Autodesk Inventor part; units mm, degrees
ref_plane "Start Plane" through (0, 0, 0) normal (0, 0, 1) x (1, 0, 0)
ref_plane "End Plane" through (0, 0, 105.4293) normal (0, 0, 1) x (1, 0, 0)
ref_plane "Work Plane4" through (163.4562, -7, -44.6771) normal (0.6544, 0, 0.7562) x (0.7562, 0, -0.6544)
ref_plane "Start Plane" through (0, 0, 0) normal (0, 0, 1) x (1, 0, 0)
ref_plane "End Plane" through (0, 0, 105.4293) normal (0, 0, 1) x (1, 0, 0)
sketch "Sketch" plane through (0, 0, 0) normal (0, 0, 1) x (1, 0, 0)
  line L0 (-10, -7) -> (-10, 7)
  line L1 (-7, 10) -> (7, 10)
  line L2 (10, 7) -> (10, -7)
  line L3 (7, -10) -> (-7, -10)
  arc A0 (-10, -7) -> (-7, -10) centre (-7, -7) ccw
  arc A1 (-7, 10) -> (-10, 7) centre (-7, 7) ccw
  arc A2 (10, 7) -> (7, 10) centre (7, 7) ccw
  arc A3 (7, -10) -> (10, -7) centre (7, -7) ccw
  arc A4 (-7, 8) -> (-8, 7) centre (-7, 7) ccw
  line L4 (-7, 8) -> (7, 8)
  arc A5 (8, 7) -> (7, 8) centre (7, 7) ccw
  line L5 (8, 7) -> (8, -7)
  arc A6 (7, -8) -> (8, -7) centre (7, -7) ccw
  line L6 (7, -8) -> (-7, -8)
  arc A7 (-8, -7) -> (-7, -8) centre (-7, -7) ccw
  line L7 (-8, -7) -> (-8, 7)
  line L8 (0, 14.8698) -> (0, -14.8698) construction
  line L9 (-14.8698, 0) -> (14.8698, 0) construction
  dimension "d7" = 3
  dimension "d10" = 20
  dimension "d11" = 20
  dimension "d12" = 2
  dimension "d15" = 10
  dimension "d16" = 10
extrude "Body" add sketch "Sketch" along normal up to surface (105.4293 mm away) from surface at 0
sketch "Sketch3" plane through (0, 0, 0) normal (0, 0, 1) x (1, 0, 0)
  line L0 (0, 0) -> (10, 0)
ref_plane "Work Plane3" through (0, 0, 0) normal (0, -1, 0) x (1, 0, 0)
sketch "Sketch4" plane through (0, 0, 0) normal (0, -1, 0) x (1, 0, 0)
  line L0 (-2, 0) -> (12, 0)
  line L1 (-2, 105.4293) -> (12, 105.4293)
  dimension "d18" = 105.4293
ref_plane "Work Plane4" through (163.4562, -7, -44.6771) normal (0.6544, 0, 0.7562) x (0.7562, 0, -0.6544)
split "Split1" plane through (163.4562, -7, -44.6771) removes the side toward (0.6544, 0, 0.7562)
sketch "Sketch9" plane through (-7, 10, 0) normal (0, 1, 0) x (1, 0, 0)
  line L0 (0, -102.8331) -> (-3, -105.4293)
  line L1 (-3, 0) -> (-3, -105.4293)
  line L2 (0, -102.8331) -> (14, -90.7177)
  line L3 (17, -88.1216) -> (14, -90.7177)
  line L4 (17, 0) -> (17, -88.1216)
  line L5 (0, 0) -> (14, 0)
  line L6 (0, 0) -> (-3, 0)
  line L7 (17, 0) -> (14, 0)
  line L8 (0.3719, -13.6065) -> (0.3719, -23.9385)
  line L9 (13.8719, -23.9385) -> (13.8719, -13.6065)
  circle A0 centre (7.1219, -18.7725) radius 8.5
  line L10 (14.1439, -13.9827) -> (14.1439, -23.5624)
  line L11 (0.2439, -23.7668) -> (0.2439, -13.7783)
  line L12 (14.1439, -13.9827) -> (14.1439, 0)
  line L13 (0.2439, -13.7783) -> (0.2439, 0)
  line L14 (17, 0) -> (17, -88.1216)
  line L15 (17, -67.4293) -> (-3, -67.4293)
  line L16 (-3, 0) -> (-3, -105.4293)
  line L17 (17, -86.1216) -> (-3, -86.1216)
  line L18 (14.1439, -23.5624) -> (14.1439, -27.2725)
  line L19 (14.1439, -27.2725) -> (0.2439, -27.2725)
  line L20 (0.2439, -27.2725) -> (0.2439, -23.7668)
  line L21 (17, -8) -> (-3, -8)
  point P0 (7, 0)
  point P1 (7.117, -27.2725)
  point P2 (14.1439, -7.7933)
  point P3 (17, -67.4293)
  point P4 (-3, -67.4293)
  point P5 (0.2439, -7.7933)
  point P6 (7.1219, -27.2725)
  point P7 (0.2439, -8)
  point P8 (14.1439, -8)
  point P9 (14.1439, -8)
  point P10 (0.2439, -8)
  dimension "d44" = 13.5
  dimension "d45" = 13.9
  dimension "d47" = 2
  dimension "d49" = 38
  dimension "d53" = 8
extrude "Extrusion8" cut sketch "Sketch9" against normal through all contours L1 L6 L5 L13 L21 | L21 L12 A0 L13 | L13 L5 L7 L12 L21 | L21 L12 L7 L4 | A0 L8 L11 | A0 L9 L8 | A0 L19 L20 | L10 A0 L9 | L18 L19 A0
equation "\"d7\" = G_IR"
equation "\"d10\" = G_H"
equation "\"d11\" = G_W"
equation "\"d12\" = G_T"
equation "\"d15\" = 0.5 * d10"
equation "\"d16\" = 0.5 * d11"
equation "\"d3\" = G_L"
equation "\"G_W\" = 20"
equation "\"G_H\" = 20"
equation "\"G_T\" = 2"
equation "\"G_IR\" = 3"
equation "\"G_L\" = d18"
equation "\"G_OFFSET_START\" = 0"
equation "\"G_OFFSET_END\" = -4.57072"
equation "\"d14\" = G_OFFSET_END + B_L"
properties part number "ISO 12633-2 - 20x20x2 - 105,43" material "Steel, Mild"
Source: CAD feature listing. Evaluate the final solid. Frame: model axes, mm. A direction names the side the tool comes from. Coordinates: 2 decimals unless noted, no trailing zeros. Loops run counter-clockwise (first coordinate to the right, second up) from the corner with the lowest first, then second, coordinate; pieces in that order, holes last. Notation, with made-up numbers: (80.5, 84.25) -> (93.5, 84.25) arc R17 ccw to (93.5, 116.25) -> close; hole circle Ø9 at (80.25, 12.5). An arc over 180 degrees is marked (long way). Answer in a Markdown table with one row per item. Add a question column.
Q1. Ray query, line 1 along Y through (x, z) = (-6.75, 80); line 2 along Y through (x, z) = (-7.5, 55). Return the intervals inside material, ascending.
Q2. Section A-A on y = -3. Return the cut outline in (x, z), and give its area (3 significant figures).
Q3. Contact query for flat-ended pins moving along their axis: pin 1 Ø1.6 at (y, z) = (9.5, 15.5) entering from -X; pin 2 Ø1 at (y, z) = (-9, 19) entering from -X; pin 3 Ø0.6 at (y, z) = (8.5, 22) entering from +X. Output: stop coordinate, or through.
Q4. Pull-direction query (X, two-part tool) for faces 4 (the face through (8, 0, 48)), 5 (the face through (9.1, 9.14, 48.78)), 6 (the face through (9, 0, 8)); classes: pulls with the +X half, pulls with the -X half, needs draft (parallel to the pull), parting line crosses it, or undercut.
Q5. Section D-D on z = 92.5. Return the cut outline in (x, y).
Q6. Section C-C on x = 2.25. Return the cut outline in (y, z), and give its area (3 significant figures).
Q7. Section B-B on z = 80. Return the cut outline in (x, y).
Q8. Reachability of faces 1 (the face through (0, -8, 65)), 2 (the face through (-9.14, 9.1, 56.03)), 3 (the face through (7.144, 9, 18)) from +Z, -Z, +X, -X, +Y, -Y: full face, straight path, thin tool, end or side. Return the list, or none.
Computed values:
| question | item | result |
|---|---|---|
| 1 | line 1 | y = -10 to -8, 8 to 10 |
| 1 | line 2 | y = -9.96 to -7.87, 7.87 to 9.96 |
| 2 | outline | (-10, 8) -> (-8, 8) -> (-8, 103.7) -> (-10, 105.43) -> close; (8, 8) -> (10, 8) -> (10, 88.12) -> (8, 89.85) -> close |
| 2 | area | 355 mm^2 |
| 3 | pin 1 | stops at x = -9.47 |
| 3 | pin 2 | stops at x = -9.6 |
| 3 | pin 3 | stops at x = 9.75 |
| 4 | face 4 | undercut |
| 4 | face 5 | pulls with the +X half |
| 4 | face 6 | needs draft |
| 5 | outline | (-10, -7) arc R3 ccw to (-7, -10) -> (4.94, -10) -> (4.94, -8) -> (-7, -8) arc R1 cw to (-8, -7) -> (-8, 7) arc R1 cw to (-7, 8) -> (4.94, 8) -> (4.94, 10) -> (-7, 10) arc R3 ccw to (-10, 7) -> close |
| 6 | outline | (-10, 27.27) -> (-8, 27.27) -> (-8, 94.83) -> (-10, 94.83) -> close; (8, 27.27) -> (10, 27.27) -> (10, 94.83) -> (8, 94.83) -> close |
| 6 | area | 270 mm^2 |
| 7 | outline | (-10, -7) arc R3 ccw to (-7, -10) -> (7, -10) arc R3 ccw to (10, -7) -> (10, 7) arc R3 ccw to (7, 10) -> (-7, 10) arc R3 ccw to (-10, 7) -> close; hole (-8, -7) arc R1 ccw to (-7, -8) -> (7, -8) arc R1 ccw to (8, -7) -> (8, 7) arc R1 ccw to (7, 8) -> (-7, 8) arc R1 ccw to (-8, 7) -> close |
| 8 | face 1 | +Z, -Z |
| 8 | face 2 | +Z, -Z, -X, +Y |
| 8 | face 3 | -Z, +Y, -Y |
